Verification items for the finished model (mm, model axes). A direction names the side the tool comes from. Round coordinates to 2 decimals unless told otherwise and drop trailing zeros. Loops run counter-clockwise (first coordinate to the right, second up) from the corner with the lowest first, then second, coordinate; pieces in that order, holes last. Notation, with made-up numbers: M -32.75,-12 L -17.75,-12 A30 ccw -17.75,21 Z; hole C -29,-39.5 d4. An arc over 180 degrees is marked long. Write item = value, one per line. Start each with the question number.
from build123d import *

# Parameters (mm, degrees)
F0_R     = 3.175
F1_DEPTH = 3.175
F2_W     = 63.5
F2_H     = 4.191
F3_DEPTH = 25.4
F4_R     = 3.175
F5_DEPTH = 25.4
F6_R     = 6.35


with BuildPart() as f1:
    # F0 (on Right) → F1 (new body)
    with BuildSketch(Plane.YZ):
        with BuildLine():
            ThreePointArc((-17.731718, 18.103163), (-17.947804, 19.309376), (-18.70349, 20.274041))
            ThreePointArc((-18.70349, 20.274041), (-27.274694, 22.950849), (-32.858508, 15.918648))
            Line((-32.858508, 15.918648), (-32.858508, -57.660647))
            Line((-32.858508, -57.660647), (30.641492, -57.660647))
            Line((30.641492, -57.660647), (30.641492, -44.960647))
            Line((30.641492, -44.960647), (-14.967139, 7.123187))
            ThreePointArc((-14.967139, 7.123187), (-20.344879, 7.203814), (-20.701, 12.570355))
            Line((-20.701, 12.570355), (-17.731718, 18.103163))
        make_face()
        with Locations((-24.940386, -35.435647)):
            Circle(F0_R, mode=Mode.SUBTRACT)
        with Locations((6.809614, -35.435647)):
            Circle(F0_R, mode=Mode.SUBTRACT)
        with Locations((-24.940386, -3.685647)):
            Circle(F0_R, mode=Mode.SUBTRACT)
    extrude(amount=F1_DEPTH)

    # F2 (on face) → F3 (join)
    with BuildSketch(Plane.YZ.offset(3.175)):
        with Locations((-1.108508, -55.565147)):
            Rectangle(F2_W, F2_H)
    extrude(amount=F3_DEPTH)

    # F4 (on face) → F5 (cut)
    with BuildSketch(Plane.XY.offset(-53.469647)):
        with Locations((17.462499, -23.333508)):
            Circle(F4_R)
        with Locations((17.462499, 21.116492)):
            Circle(F4_R)
        with Locations((12.1285, -2.161645)):
            Circle(F4_R)
    extrude(amount=-F5_DEPTH, mode=Mode.SUBTRACT)

    # F6
    f6_edges = [f1.edges().sort_by_distance(p)[0] for p in [
        (3.175, -1.108508, -53.469647),
        (0, -1.108508, -57.660647),
    ]]
    fillet(f6_edges, radius=F6_R)


solid = f1.part
1. Section check C-C, the plane z = -2.5. Enter the section's corners in (x, y) (1 decimal).
2. Section check A-A, the plane x = 13. Enter the section's corners in (y, z).
3. Section check D-D, the plane x = 18.25. Enter the section's corners in (y, z), and give its area (3 significant figures).
4. Section check B-B, the plane y = 22. Enter the section's corners in (x, z) (3 decimals).
5. Gauge pin test, flat ends, axial feed: P1, Ø15, axis at x = 21, y = -8.5, coming from the +Z side; P2, Ø8.5, axis at x = 12.13, y = -2.16, coming from the +Z side. Record the tip position at first contact, or that the pin passes through.
6. Mould release check, pull along Z, two halves, no side actions. Record for faces 1 (the cylindrical face through (1.81, -0.66, -55.75)), 2 (the cylindrical face through (5.085, 15.365, -51.659)), 3 (the cylindrical face through (1.57, 8.52, -32.76)), 4 (the flat face through (0, -9, -22)): pulls with the +Z half, pulls with the -Z half, needs draft (parallel to the pull), parting line crosses it, or undercut.
7. Tool access check on faces 5 (the flat face through (19, -2, -53.47)), 6 (the cylindrical face through (17.049, 24.264, -55.536)), 7 (the flat face through (1.565, -19.237, 15.298)). Record the directions out of +Z, -Z, +X, -X, +Y, -Y that give a thin tool (end or side, any length) a straight path to the whole face; none if there is none.
8. Thickness scan on line 1 (Z direction, x = 15.75, y = 0.5); line 2 (X direction, y = -29, z = -24) (3 decimals); line 3 (X direction, y = -8.5, z = -52). Record the ranges inside material, lowest first.
Computed values:
q1.outline = M 0,-32.9 L 3.2,-32.9 L 3.2,-27.9 L 0,-27.9 Z; M 0,-22 L 3.2,-22 L 3.2,-6.5 L 0,-6.5 Z
q2.outline = M -32.86,-57.66 L -5.21,-57.66 L -5.21,-53.47 L -32.86,-53.47 Z; M 0.89,-57.66 L 30.64,-57.66 L 30.64,-53.47 L 0.89,-53.47 Z
q3.outline = M -32.86,-57.66 L -26.41,-57.66 L -26.41,-53.47 L -32.86,-53.47 Z; M -20.26,-57.66 L 18.04,-57.66 L 18.04,-53.47 L -20.26,-53.47 Z; M 24.19,-57.66 L 30.64,-57.66 L 30.64,-53.47 L 24.19,-53.47 Z
q3.area = 215 mm2
q4.outline = M 0,-51.311 A6.35 ccw 6.35,-57.661 L 14.413,-57.661 L 14.413,-53.47 L 9.525,-53.47 A6.35 cw 3.175,-47.12 L 3.175,-35.092 L 0,-35.092 Z; M 20.512,-57.661 L 28.575,-57.661 L 28.575,-53.47 L 20.512,-53.47 Z
q5.P1 = -53.47
q5.P2 = -53.28
q6.face_1 = pulls with the -Z half
q6.face_2 = pulls with the +Z half
q6.face_3 = undercut
q6.face_4 = needs draft
q7.face_5 = +Z, +X, +Y, -Y
q7.face_6 = +Z, -Z
q7.face_7 = +X, -X, +Y
q8.line_1 = -57.66 to -53.47
q8.line_2 = 0 to 3.175
q8.line_3 = 0.04 to 5.46
